Input: part model. Units: mm. Frame: model coordinates. Round coordinates to 2 decimals unless told otherwise and drop trailing zeros. Write each loop counter-clockwise with the first axis right and the second up, starting at its lowest first coordinate (ties: lowest second). Pieces come first, ordered by that corner, then holes. Notation, with made-up numbers: (39, 23.5) - (49, 23.5) arc R20 cw to (49, 55.5) - close; hole circle Ø3 at (81.5, 5). An arc over 180 degrees is marked (long way). Use one line per item in the form item = value.
Autodesk Inventor part; units mm, degrees
ref_plane "YZ Plane" through (0, 0, 0) normal (1, 0, 0) x (0, 1, 0)
ref_plane "XZ Plane" through (0, 0, 0) normal (0, 1, 0) x (-1, 0, 0)
ref_plane "XY Plane" through (0, 0, 0) normal (0, 0, 1) x (1, 0, 0)
sketch "Sketch1" plane through (0, 0, 0) normal (0, 0, 1) x (1, 0, 0)
  line L0 (0, 0) -> (152.4, 0)
  line L1 (152.4, 0) -> (152.4, 101.6)
  line L2 (152.4, 101.6) -> (0, 101.6)
  line L3 (0, 101.6) -> (0, 0)
  dimension "d0" = 152.4
  dimension "d1" = 101.6
extrude "Extrusion1" add sketch "Sketch1" along normal blind 4.7625
sketch "Sketch2" plane through (0, 0, 4.7625) normal (0, 0, 1) x (1, 0, 0)
  line L0 (0, 0) -> (0, 101.6)
  line L1 (0, 101.6) -> (152.4, 101.6)
  circle A0 centre (76.2, 88.9) radius 4.7625
  dimension "d4" = 76.2
  dimension "d5" = 12.7
  dimension "d25" = 9.525
extrude "Extrusion2" cut sketch "Sketch2" against normal up to next
sketch "Sketch3" plane through (0, 0, 4.7625) normal (0, 0, 1) x (1, 0, 0)
  line L0 (0, 0) -> (0, 101.6)
  line L1 (152.4, 0) -> (0, 0)
  circle A0 centre (12.7, 12.7) radius 2.3813
  dimension "d8" = 4.7625
  dimension "d9" = 12.7
  dimension "d10" = 12.7
extrude "Extrusion3" cut sketch "Sketch3" against normal up to next
pattern_linear "Rectangular Pattern1" count 6 spacing 25.4 along (1, 0, 0) count 2 spacing 25.4 along (0, 1, 0) of "Extrusion3"
sketch "Sketch4" plane through (0, 0, 4.7625) normal (0, 0, 1) x (1, 0, 0)
  line L0 (0, 0) -> (0, 101.6)
  line L1 (152.4, 101.6) -> (152.4, 0)
  line L2 (0, 101.6) -> (152.4, 101.6)
  line L3 (0, 50.8) -> (63.5, 101.6)
  line L4 (0, 101.6) -> (0, 50.8)
  line L5 (63.5, 101.6) -> (0, 101.6)
  line L6 (152.4, 101.6) -> (152.4, 50.8)
  line L7 (88.9, 101.6) -> (152.4, 50.8)
  line L8 (152.4, 101.6) -> (88.9, 101.6)
  dimension "d19" = 63.5
  dimension "d20" = 63.5
  dimension "d21" = 50.8
extrude "Extrusion4" cut sketch "Sketch4" against normal up to next
fillet "Fillet1" radius 3.175 6 edges at (63.5, 101.6, 2.3813) (88.9, 101.6, 2.3813) (152.4, 50.8, 2.3813) (152.4, 0, 2.3813) (0, 0, 2.3813) (0, 50.8, 2.3813)
properties part number "Frame_MidRollerPlate" material "Aluminum-6061"
(1) Draft query along X for faces 1 (the face through (87.01, 36.65, 2.41)), 2 (the face through (152.4, 26, 2)), 3 (the face through (0.91, 0.95, 2.41)). Return one class per face: released by +X, released by -X, zero draft, split by the parting line, or undercut.
Derived:
face_1 = undercut
face_2 = released by +X
face_3 = released by -X
(2) Cut plane C-C on z = 3.5. Count the separate pieces of the cut face and the enclosed holes in it, then the cut area to 3 significant figures.
Derived:
separate_pieces = 1
enclosed_holes = 13
area = 12,000 mm^2
(3) Cut plane D-D on x = 76.2. Output: boundary loops of the cut face in (y, z), then the cut area to 3 significant figures.
Derived:
outline = (0, 0) - (84.14, 0) - (84.14, 4.76) - (0, 4.76) - close; (93.66, 0) - (101.6, 0) - (101.6, 4.76) - (93.66, 4.76) - close
area = 439 mm^2
(4) Material intervals for L1, parallel to Y at x = 114, z = 3.85; L2, parallel to Y at x = 38.1, z = 3.55; L3, parallel to Y at x = 73, z = 1.6, sorted ascending.
Derived:
L1 = 0 to 10.34, 15.06 to 35.74, 40.46 to 81.52
L2 = 0 to 10.32, 15.08 to 35.72, 40.48 to 81.28
L3 = 0 to 85.37, 92.43 to 101.6
(5) First-contact query: pin 1 Ø5.5 at (x, y) = (12.7, 38.1) entering from +Z; pin 2 Ø1.5 at (y, z) = (87.5, 3) entering from +X. Flat tips, straight axial feed; report the tip coordinate or a pass-through.
Derived:
pin_1 = 4.76
pin_2 = 107.46
(6) Cut plane B-B on y = 12.7. Output: boundary loops of the cut face in (x, z).
Derived:
outline = (0, 0) - (10.32, 0) - (10.32, 4.76) - (0, 4.76) - close; (15.08, 0) - (35.72, 0) - (35.72, 4.76) - (15.08, 4.76) - close; (40.48, 0) - (61.12, 0) - (61.12, 4.76) - (40.48, 4.76) - close; (65.88, 0) - (86.52, 0) - (86.52, 4.76) - (65.88, 4.76) - close; (91.28, 0) - (111.92, 0) - (111.92, 4.76) - (91.28, 4.76) - close; (116.68, 0) - (137.32, 0) - (137.32, 4.76) - (116.68, 4.76) - close; (142.08, 0) - (152.4, 0) - (152.4, 4.76) - (142.08, 4.76) - close
(7) Cut plane A-A on x = 12.7. Output: boundary loops of the cut face in (y, z), then the cut area to 3 significant figures.
Derived:
outline = (0, 0) - (10.32, 0) - (10.32, 4.76) - (0, 4.76) - close; (15.08, 0) - (35.72, 0) - (35.72, 4.76) - (15.08, 4.76) - close; (40.48, 0) - (60.96, 0) - (60.96, 4.76) - (40.48, 4.76) - close
area = 245 mm^2
